Verification items for this drawing (mm, ordinates from the low corner). A direction names the side the tool comes from. Round coordinates to 2 decimals unless told otherwise and drop trailing zeros. Write each loop counter-clockwise with the first axis right and the second up, starting at its lowest first coordinate (ties: lowest second). Pieces come first, ordered by that corner, then holes. Notation, with made-up numbers: M -12,-31.75 L 34,-31.75 A19 cw 34,-8.75 Z; hole C -12.5,0.5 d10. An arc over 180 degrees is marked long. One line per question, with ' | ' between items. Start each with the question number.
Q1. Cross-section at B-B (y = 19.5). Record the boundary of the cut face in (x, z), then the cut area to 3 significant figures.
Q2. Tool access check on the marked faces 3 and 4. Record the directions out of +Z, -Z, +X, -X, +Y, -Y that give a thin tool (end or side, any length) a straight path to the whole face; none if there is none.
Q3. Cross-section at D-D (x = 57.5). Record the boundary of the cut face in (y, z).
Q4. Gauge pin test, flat ends, axial feed: pin 1 (0.8 mm diameter, centred on y = 3.5, z = 31, fed in from +X); pin 2 (1 mm diameter, centred on x = 45.5, y = 33, fed in from +Z); pin 3 (1 mm diameter, centred on y = 9, z = 51.5, fed in from +X) (1 decimal); pin 4 (4.5 mm diameter, centred on x = 30, z = 30, fed in from -Y). Record the tip position at first contact, or that the pin passes through.
Q5. Cross-section at C-C (z = 52). Record the boundary of the cut face in (x, y) (1 decimal), then the cut area to 3 significant figures.
Q6. Thickness scan on line 1 along X through (y, z) = (41.9, 30); line 2 along X through (y, z) = (2, 30). Record the ranges inside material, lowest first. Write a range as from..to.
Q7. Release check for a two-part mould opening along X. For the marked faces 1 and 2 record: released by +X, released by -X, zero draft, split by the parting line, or undercut.
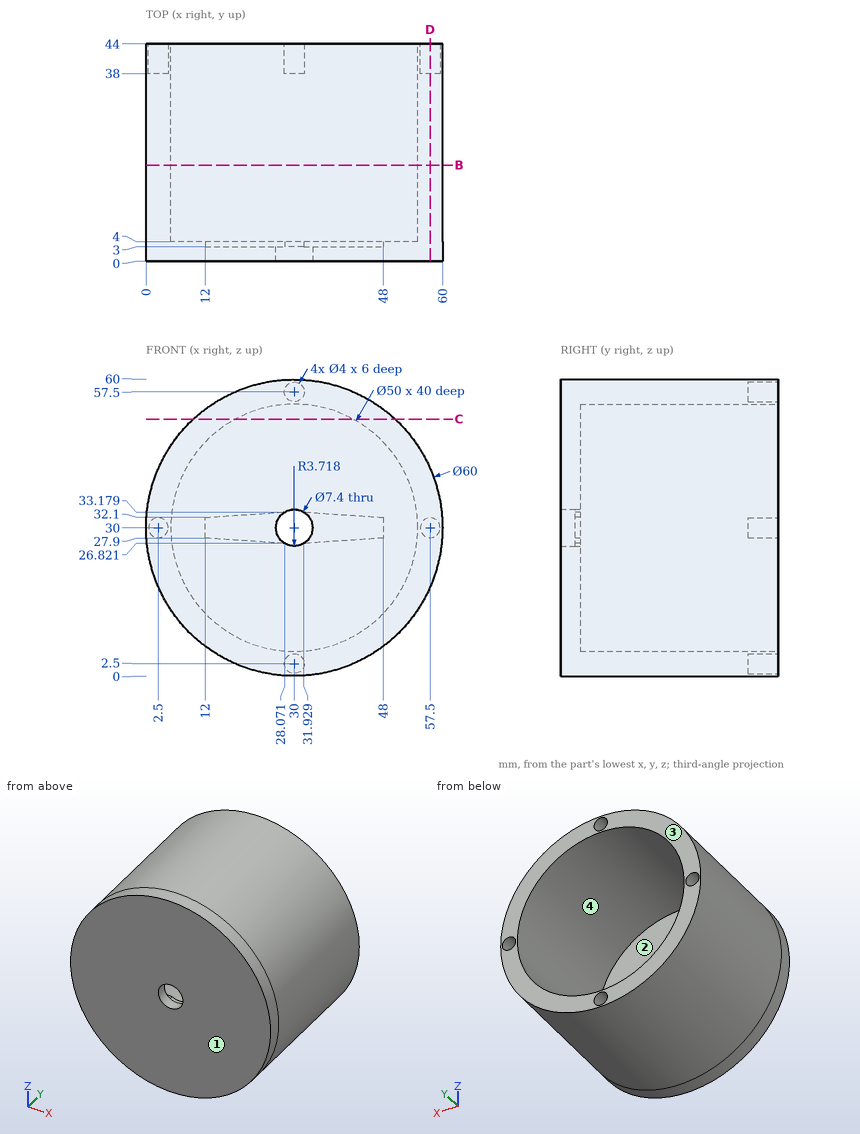
Determined:
1) outline: C 30,30 d60; hole C 30,30 d50 | area: 864 mm²
2) face 3: +Z, -Z, +X, -X, +Y | face 4: +Y
3) outline: M 0,18.01 L 44,18.01 L 44,28 L 38,28 L 38,32 L 44,32 L 44,41.99 L 0,41.99 Z
4) pin 1: stops at x = 59.99 | pin 2: stops at z = 55.98 | pin 3: stops at x = 51.4 | pin 4: passes through
5) outline: M 9.6,0 L 50.4,0 L 50.4,44 L 41.9,44 L 41.9,4 L 18.1,4 L 18.1,44 L 9.6,44 Z | area: 845 mm²
6) line 1: x = 0..0.5, 4.5..5, 55..55.5, 59.5..60 | line 2: x = 0..26.3, 33.7..60
7) face 1: zero draft | face 2: undercut
